The listing builds one solid part. Answer for the finished solid, in the listing's coordinates (mm). Coordinates: 2 decimals unless noted, no trailing zeros. Order: outer loops, then holes, each group sorted by start corner. A loop starts at its lowest first (then second) coordinate and runs counter-clockwise, first axis right, second up.
from build123d import *

# Parameters (mm, degrees)
CROQUIS2_W              = 44.460320701
CROQUIS2_H              = 20
SALIENTE_EXTRUIR2_DEPTH = 25
CROQUIS3_R              = 1.5
CORTAR_EXTRUIR1_DEPTH   = 21
CROQUIS4_R              = 1.5
CORTAR_EXTRUIR2_DEPTH   = 50


with BuildPart() as part:
    # Croquis2 → Saliente-Extruir2 (new body)
    with BuildSketch(Plane(origin=(0, 0, 0), x_dir=(0, 0, -1), z_dir=(1, 0, 0))):
        with Locations((-22.230160351, -10)):
            Rectangle(CROQUIS2_W, CROQUIS2_H)
    extrude(amount=SALIENTE_EXTRUIR2_DEPTH)

    # Croquis3 → Cortar-Extruir1 (cut, through all)
    with BuildSketch(Plane.XZ.offset(20)):
        with Locations((12.5, 10)):
            Circle(CROQUIS3_R)
        with Locations((12.5, 34.460320701)):
            Circle(CROQUIS3_R)
    extrude(amount=-CORTAR_EXTRUIR1_DEPTH, mode=Mode.SUBTRACT)

    # Croquis4 → Cortar-Extruir2 (cut)
    with BuildSketch(Plane(origin=(25, 0, 0), x_dir=(0, 0, -1), z_dir=(1, 0, 0))):
        with Locations((-29.460320701, -10)):
            Circle(CROQUIS4_R)
        with Locations((-15, -10)):
            Circle(CROQUIS4_R)
    extrude(amount=-CORTAR_EXTRUIR2_DEPTH, mode=Mode.SUBTRACT)


solid = part.part
(1) Find section C-C on y = -10. Determine the outline of the cut face in (x, z).
(2) Find the intervals of material crossed by probe 1 along Z at (x, y) = (12.5, -5.75); probe 2 along Z at (x, y) = (16.5, -11.25); probe 3 along Z at (x, y) = (12, -10.75), in increasing order.
(3) Find section D-D on x = 2. Determine the outline of the cut face in (y, z).
(4) Find section B-B on z = 15. Determine the outline of the cut face in (x, y).
(5) The mould has two halves that part along Z. Classify faces 1 (the cylindrical face through (12.175, -10.14, 32.996)), 2 (the cylindrical face through (12.68, -9.93, 30.96)), 3 (the flat face through (12, 0, 23)), 4 (the flat face through (12, -10, 44.46)): pulls with the +Z half, pulls with the -Z half, needs draft (parallel to the pull), parting line crosses it, or undercut.
(6) Given pin 1 Ø2.5 at (x, z) = (12.5, 34.46) entering from +Y, flat-ended and moving along its own axis, determine where the tip first touches the part or whether it passes through.
(7) Find section A-A on x = 12.5. Determine the outline of the cut face in (y, z), then the cut area to 3 significant figures.
Resolved:
1. outline: (0, 0) - (25, 0) - (25, 13.5) - (0, 13.5) - close; (0, 16.5) - (25, 16.5) - (25, 27.96) - (0, 27.96) - close; (0, 30.96) - (25, 30.96) - (25, 44.46) - (0, 44.46) - close; hole circle Ø3 at (12.5, 10); hole circle Ø3 at (12.5, 34.46)
2. probe 1: z = 0 to 8.5, 11.5 to 32.96, 35.96 to 44.46
2. probe 2: z = 0 to 14.17, 15.83 to 28.63, 30.29 to 44.46
2. probe 3: z = 0 to 8.59, 11.41 to 13.7, 16.3 to 28.16, 30.76 to 33.05, 35.87 to 44.46
3. outline: (-20, 0) - (0, 0) - (0, 44.46) - (-20, 44.46) - close; hole circle Ø3 at (-10, 15); hole circle Ø3 at (-10, 29.46)
4. outline: (0, -20) - (25, -20) - (25, -11.5) - (0, -11.5) - close; (0, -8.5) - (25, -8.5) - (25, 0) - (0, 0) - close
5. face 1: undercut
5. face 2: undercut
5. face 3: needs draft
5. face 4: pulls with the +Z half
6. pin 1: passes through
7. outline: (-20, 0) - (0, 0) - (0, 8.5) - (-20, 8.5) - close; (-20, 11.5) - (0, 11.5) - (0, 32.96) - (-20, 32.96) - close; (-20, 35.96) - (0, 35.96) - (0, 44.46) - (-20, 44.46) - close; hole circle Ø3 at (-10, 15); hole circle Ø3 at (-10, 29.46)
7. area: 755 mm2
